Source: CAD feature listing. Evaluate the final solid. Frame: model axes, mm. Face numbers are marked on the shaded views. A direction names the side the tool comes from. Round coordinates to 2 decimals unless told otherwise and drop trailing zeros. Write each loop counter-clockwise with the first axis right and the second up, starting at its lowest first coordinate (ties: lowest second). Pieces come first, ordered by that corner, then holes. Notation, with made-up numbers: (-17, -17.75) -> (-10, -17.75) arc R22 ccw to (-10, 12.25) -> close; hole circle Ø8 at (82, 62). An arc over 180 degrees is marked (long way). Return JSON: item names as keys, results as strings. Group by question number.
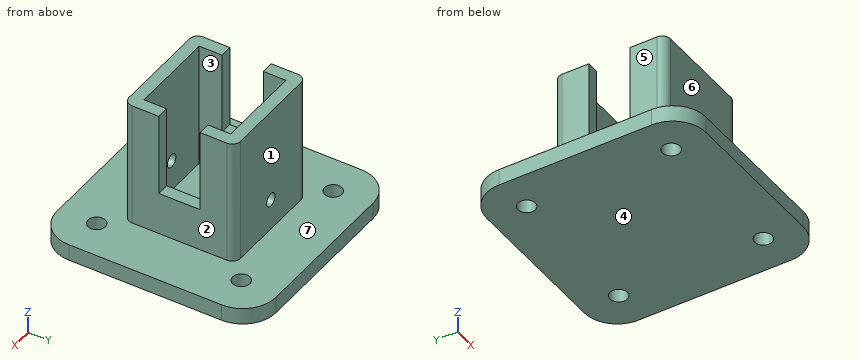
from build123d import *

# Parameters (mm, degrees)
SKETCH1_W           = 27
SKETCH1_H           = 27
SKETCH1_W_2         = 21
SKETCH1_H_2         = 21
BOSS_EXTRUDE1_DEPTH = 15.2
SKETCH2_R           = 1.6
CUT_EXTRUDE1_DEPTH  = 34.797780992
SKETCH5_R           = 2.1
SKETCH5_W           = 27
SKETCH5_H           = 27
SKETCH5_W_2         = 21
SKETCH5_H_2         = 21
BOSS_EXTRUDE3_DEPTH = 4
FILLET2_R           = 2
BOSS_EXTRUDE5_DEPTH = 4
SKETCH8_W           = 21
SKETCH8_H           = 21
BOSS_EXTRUDE7_DEPTH = 15.2
SKETCH9_W           = 20
SKETCH9_H           = 10
CUT_EXTRUDE2_DEPTH  = 57.801496459


with BuildPart() as part:
    # Sketch1 → Boss-Extrude1 (new body)
    with BuildSketch(Plane.XY):
        Rectangle(SKETCH1_W, SKETCH1_H)
        Rectangle(SKETCH1_W_2, SKETCH1_H_2, mode=Mode.SUBTRACT)
    extrude(amount=BOSS_EXTRUDE1_DEPTH)

    # Sketch2 → Cut-Extrude1 (cut, through all)
    with BuildSketch(Plane.XZ.offset(13.5)):
        with Locations((0, 7.6)):
            Circle(SKETCH2_R)
    extrude(amount=-CUT_EXTRUDE1_DEPTH, mode=Mode.SUBTRACT)

    # Sketch5 → Boss-Extrude3 (add)
    with BuildSketch(Plane(origin=(0, 0, 0), x_dir=(-1, 0, 0), z_dir=(0, 0, -1))):
        with BuildLine():
            Line((18.5, 21.5), (-18.5, 21.5))
            ThreePointArc((-18.5, 21.5), (-20.621320344, 20.621320344), (-21.5, 18.5))
            Line((-21.5, 18.5), (-21.5, -18.5))
            ThreePointArc((-21.5, -18.5), (-20.621320344, -20.621320344), (-18.5, -21.5))
            Line((-18.5, -21.5), (18.5, -21.5))
            ThreePointArc((18.5, -21.5), (20.621320344, -20.621320344), (21.5, -18.5))
            Line((21.5, -18.5), (21.5, 18.5))
            ThreePointArc((21.5, 18.5), (20.621320344, 20.621320344), (18.5, 21.5))
        make_face()
        with Locations((-17.5, 17.5)):
            Circle(SKETCH5_R, mode=Mode.SUBTRACT)
        with Locations((-17.5, -17.5)):
            Circle(SKETCH5_R, mode=Mode.SUBTRACT)
        with Locations((17.5, -17.5)):
            Circle(SKETCH5_R, mode=Mode.SUBTRACT)
        with Locations((17.5, 17.5)):
            Circle(SKETCH5_R, mode=Mode.SUBTRACT)
        Rectangle(SKETCH5_W, SKETCH5_H, mode=Mode.SUBTRACT)
        Rectangle(SKETCH5_W, SKETCH5_H)
        Rectangle(SKETCH5_W_2, SKETCH5_H_2, mode=Mode.SUBTRACT)
        Rectangle(SKETCH5_W_2, SKETCH5_H_2)
    extrude(amount=BOSS_EXTRUDE3_DEPTH)

    # Fillet2
    fillet2_edges = [part.edges().sort_by_distance(p)[0] for p in [
        (13.5, -13.5, 7.6),
        (-13.5, -13.5, 7.6),
        (-13.5, 13.5, 7.6),
        (13.5, 13.5, 7.6),
    ]]
    fillet(fillet2_edges, radius=FILLET2_R)

    # Sketch7 → Boss-Extrude5 (add)
    with BuildSketch(Plane.XY):
        with BuildLine():
            Line((18.5, 26.5), (-18.5, 26.5))
            ThreePointArc((-18.5, 26.5), (-24.156854249, 24.156854249), (-26.5, 18.5))
            Line((-26.5, 18.5), (-26.5, -18.5))
            ThreePointArc((-26.5, -18.5), (-24.156854249, -24.156854249), (-18.5, -26.5))
            Line((-18.5, -26.5), (18.5, -26.5))
            ThreePointArc((18.5, -26.5), (24.156854249, -24.156854249), (26.5, -18.5))
            Line((26.5, -18.5), (26.5, 18.5))
            ThreePointArc((26.5, 18.5), (24.156854249, 24.156854249), (18.5, 26.5))
        make_face()
        with BuildLine():
            Line((18.5, 21.5), (-18.5, 21.5))
            ThreePointArc((-18.5, 21.5), (-20.621320344, 20.621320344), (-21.5, 18.5))
            Line((-21.5, 18.5), (-21.5, -18.5))
            ThreePointArc((-21.5, -18.5), (-20.621320344, -20.621320344), (-18.5, -21.5))
            Line((-18.5, -21.5), (18.5, -21.5))
            ThreePointArc((18.5, -21.5), (20.621320344, -20.621320344), (21.5, -18.5))
            Line((21.5, -18.5), (21.5, 18.5))
            ThreePointArc((21.5, 18.5), (20.621320344, 20.621320344), (18.5, 21.5))
        make_face(mode=Mode.SUBTRACT)
    extrude(amount=-BOSS_EXTRUDE5_DEPTH)

    # Sketch8 → Boss-Extrude7 (add)
    with BuildSketch(Plane.XY.offset(15.2)):
        with BuildLine():
            ThreePointArc((-11.5, 13.5), (-12.914213562, 12.914213562), (-13.5, 11.5))
            Line((-13.5, 11.5), (-13.5, -11.5))
            ThreePointArc((-13.5, -11.5), (-12.914213562, -12.914213562), (-11.5, -13.5))
            Line((-11.5, -13.5), (11.5, -13.5))
            ThreePointArc((11.5, -13.5), (12.914213562, -12.914213562), (13.5, -11.5))
            Line((13.5, -11.5), (13.5, 11.5))
            ThreePointArc((13.5, 11.5), (12.914213562, 12.914213562), (11.5, 13.5))
            Line((11.5, 13.5), (-11.5, 13.5))
        make_face()
        Rectangle(SKETCH8_W, SKETCH8_H, mode=Mode.SUBTRACT)
    extrude(amount=BOSS_EXTRUDE7_DEPTH)

    # Sketch9 → Cut-Extrude2 (cut, through all)
    with BuildSketch(Plane(origin=(13.5, 0, 0), x_dir=(0, 0, -1), z_dir=(1, 0, 0))):
        with Locations((-20.4, 0)):
            Rectangle(SKETCH9_W, SKETCH9_H)
    extrude(amount=-CUT_EXTRUDE2_DEPTH, mode=Mode.SUBTRACT)


solid = part.part
Item 1: Material intervals for probe 1 along Y at (x, z) = (-17.5, -1.9); probe 2 along Y at (x, z) = (-8.5, 20.5), sorted ascending.
Item 2: Cut plane A-A on x = 17.5. Output: boundary loops of the cut face in (y, z).
Item 3: Set-up query: the marked faces 4, 5, 6 and 7. Return all of +Z, -Z, +X, -X, +Y, -Y with unobstructed straight access to the full face (end or side cutting, diameter ignored); none if empty.
Item 4: Pull-direction query (Y, two-part tool) for the marked faces 1, 2 and 3; classes: +Y half, -Y half, draft (parallel to the pull), parting line (faces both ways), or undercut.
Item 5: First-contact query: pin 1 Ø2.5 at (x, y) = (-17.5, 17.5) entering from +Z; pin 2 Ø12 at (x, y) = (-12.5, -14.5) entering from +Z; pin 3 Ø1.5 at (x, z) = (11.5, 21.5) entering from +Y; pin 4 Ø5.5 at (x, y) = (-17.5, -17.5) entering from +Z. Flat tips, straight axial feed; report the tip coordinate or a pass-through.
Item 6: Cut plane D-D on y = 2. Output: boundary loops of the cut face in (x, z).
Item 7: Cut plane C-C on z = 7.6. Output: boundary loops of the cut face in (x, y).
Here are the results:
{
 "1": {"probe 1": "y = -26.5 to -19.6, -15.4 to 15.4, 19.6 to 26.5", "probe 2": "y = -13.5 to -10.5, 10.5 to 13.5"},
 "2": {"outline": "(-26.5, -4) -> (-19.6, -4) -> (-19.6, 0) -> (-26.5, 0) -> close; (-15.4, -4) -> (15.4, -4) -> (15.4, 0) -> (-15.4, 0) -> close; (19.6, -4) -> (26.5, -4) -> (26.5, 0) -> (19.6, 0) -> close"},
 "3": {"face 4": "-Z, +X, -X, +Y, -Y", "face 5": "+Z, -X, +Y, -Y", "face 6": "+Z, +X, -X, -Y", "face 7": "+Z"},
 "4": {"face 1": "+Y half", "face 2": "draft", "face 3": "undercut"},
 "5": {"pin 1": "passes through", "pin 2": "stops at z = 30.4", "pin 3": "stops at y = 13.5", "pin 4": "stops at z = 0"},
 "6": {"outline": "(-26.5, -4) -> (26.5, -4) -> (26.5, 0) -> (13.5, 0) -> (13.5, 10.4) -> (10.5, 10.4) -> (10.5, 0) -> (-10.5, 0) -> (-10.5, 10.4) -> (-13.5, 10.4) -> (-13.5, 0) -> (-26.5, 0) -> close"},
 "7": {"outline": "(-13.5, -11.5) arc R2 ccw to (-11.5, -13.5) -> (-1.6, -13.5) -> (-1.6, -10.5) -> (-10.5, -10.5) -> (-10.5, 10.5) -> (-1.6, 10.5) -> (-1.6, 13.5) -> (-11.5, 13.5) arc R2 ccw to (-13.5, 11.5) -> close; (1.6, -13.5) -> (11.5, -13.5) arc R2 ccw to (13.5, -11.5) -> (13.5, 11.5) arc R2 ccw to (11.5, 13.5) -> (1.6, 13.5) -> (1.6, 10.5) -> (10.5, 10.5) -> (10.5, -10.5) -> (1.6, -10.5) -> close"}
}
